Can you work these out from the model? Positions are in its coordinate system, mm. Face numbers are marked on the shaded views. Give positions to 0.01 mm unless a question says otherwise; leave off trailing zeros. Write each loop counter-clockwise with the first axis right and the second up, starting at its lowest first coordinate (ties: lowest second). Pieces come first, ordered by that corner, then holes. Notation, with made-up numbers: (-20.5, 64) -> (22.5, 64) arc R27 cw to (22.5, 102) -> close; hole circle Ø9 at (-18, -18). An arc over 180 degrees is marked (long way). Answer as CSV lines item,"result". Start each with the question number.
1. I'm going to push flat-ended pins straight in: P1, Ø1, axis at y = -1.5, z = -4, coming from the +X side; P2, Ø2.5, axis at x = 7, y = -5.5, coming from the +Z side. Where does each tip first touch, or does it pass through?
2. If we section it at D-D on x = 8.5: Write out the boundary of the cut face in (y, z), plus the area to 3 significant figures.
3. If we section it at A-A on z = -13: Write out the boundary of the cut face in (x, y).
4. If we section it at B-B on x = -6.5: Write out the boundary of the cut face in (y, z).
5. If we mould it in two halves opening along Y, with no side actions, what happens to the marked faces 1, 2, 3 and 4? For each: pulls with the +Y half, pulls with the -Y half, needs draft (parallel to the pull), parting line crosses it, or undercut.
6. I need wall thicknesses on line 1 (Z direction, x = -4.5, y = -2.5); line 2 (Z direction, x = -1.75, y = -1.25); line 3 (X direction, y = -7.25, z = 10). Which ranges of each line are inside material? Lowest first, please. Write a range as [from, to].
7. If we section it at C-C on x = 2.75: Write out the boundary of the cut face in (y, z).
```python
from build123d import *

# Parameters (mm, degrees)
F0_W      = 22.75429
F0_H      = 42.548669
F1_DEPTH  = 9.398
F2_R      = 2.54
F4_DEPTH  = 0.508
F6_DEPTH  = 1.9812
F7_R      = 3.013325
F8_DEPTH  = 1.9812
F9_R      = 2.713026
F10_DEPTH = 1.0414
F11_R     = 1.117074
F12_DEPTH = 0.5588
F13_R     = 2.450394
F14_DEPTH = 1.1176
F15_R     = 1.193925
F16_DEPTH = 0.6604


with BuildPart() as f1:
    # F0 (on Front) → F1 (new body)
    with BuildSketch(Plane.XZ):
        with Locations((1.757446, -0.647479)):
            Rectangle(F0_W, F0_H)
    extrude(amount=F1_DEPTH)

    # F2
    f2_edges = [f1.edges().sort_by_distance(p)[0] for p in [
        (13.134591, -9.398, -0.647479),
        (-9.619699, -9.398, -0.647479),
        (13.134591, 0, -0.647479),
        (-9.619699, 0, -0.647479),
    ]]
    fillet(f2_edges, radius=F2_R)

    # F3 (on face) → F4 (cut)
    with BuildSketch(Plane.XY.offset(20.626856)):
        with BuildLine():
            Line((9.49368, -0.802048), (-5.928423, -0.802048))
            ThreePointArc((-5.928423, -0.802048), (-7.724474, -1.545997), (-8.468423, -3.342048))
            Line((-8.468423, -3.342048), (-8.468423, -6.049972))
            ThreePointArc((-8.468423, -6.049972), (-7.724474, -7.846024), (-5.928423, -8.589972))
            Line((-5.928423, -8.589972), (9.49368, -8.589972))
            ThreePointArc((9.49368, -8.589972), (11.289732, -7.846024), (12.03368, -6.049972))
            Line((12.03368, -6.049972), (12.03368, -3.342048))
            ThreePointArc((12.03368, -3.342048), (11.289732, -1.545997), (9.49368, -0.802048))
        make_face()
    extrude(amount=-F4_DEPTH, mode=Mode.SUBTRACT)

    # F5 (on face) → F6 (join)
    with BuildSketch(Plane.XY.offset(20.118856)):
        Polygon((9.422873, -2.225276), (6.099785, -2.225276), (4.438241, -5.103154), (6.099785, -7.981033), (9.422873, -7.981033), (11.084417, -5.103154), align=None)
    extrude(amount=F6_DEPTH)

    # F7 (on face) → F8 (join)
    with BuildSketch(Plane.XY.offset(20.118856)):
        with Locations((-4.526955, -4.731211)):
            Circle(F7_R)
    extrude(amount=F8_DEPTH)

    # F9 (on face) → F10 (cut)
    with BuildSketch(Plane.XY.offset(22.100056)):
        with Locations((-4.526955, -4.731211)):
            Circle(F9_R)
    extrude(amount=-F10_DEPTH, mode=Mode.SUBTRACT)

    # F11 (on face) → F12 (join)
    with BuildSketch(Plane.XY.offset(21.058656)):
        with Locations((-4.526955, -4.731211)):
            Circle(F11_R)
    extrude(amount=F12_DEPTH)

    # F13 (on face) → F14 (cut)
    with BuildSketch(Plane.XY.offset(22.100056)):
        with Locations((7.78931, -5.203744)):
            Circle(F13_R)
    extrude(amount=-F14_DEPTH, mode=Mode.SUBTRACT)

    # F15 (on face) → F16 (join)
    with BuildSketch(Plane.XY.offset(20.982456)):
        with Locations((7.78931, -5.203744)):
            Circle(F15_R)
    extrude(amount=F16_DEPTH)


solid = f1.part
```
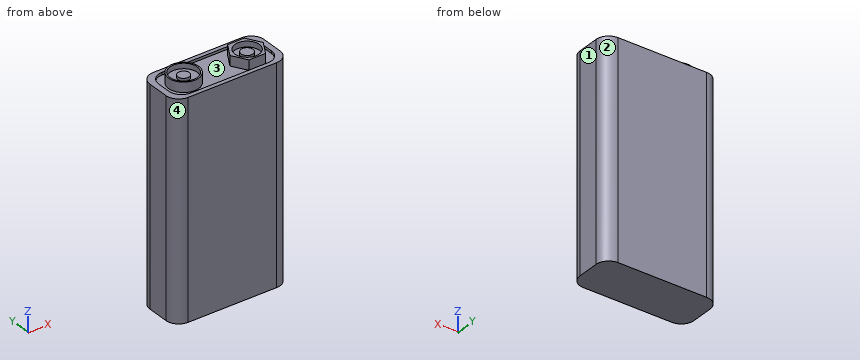
Computed values:
1,P1,"stops at x = 13.08"
1,P2,"stops at z = 21.64"
2,outline,"(-9.4, -21.92) -> (0, -21.92) -> (0, 20.63) -> (-0.8, 20.63) -> (-0.8, 20.12) -> (-2.23, 20.12) -> (-2.23, 22.1) -> (-2.86, 22.1) -> (-2.86, 20.98) -> (-4.24, 20.98) -> (-4.24, 21.64) -> (-6.16, 21.64) -> (-6.16, 20.98) -> (-7.55, 20.98) -> (-7.55, 22.1) -> (-7.98, 22.1) -> (-7.98, 20.12) -> (-8.59, 20.12) -> (-8.59, 20.63) -> (-9.4, 20.63) -> close"
2,area,"403 mm2"
3,outline,"(-9.62, -6.86) arc R2.54 ccw to (-7.08, -9.4) -> (10.59, -9.4) arc R2.54 ccw to (13.13, -6.86) -> (13.13, -2.54) arc R2.54 ccw to (10.59, 0) -> (-7.08, 0) arc R2.54 ccw to (-9.62, -2.54) -> close"
4,outline,"(-9.4, -21.92) -> (0, -21.92) -> (0, 20.63) -> (-0.87, 20.63) -> (-0.87, 20.12) -> (-2.45, 20.12) -> (-2.45, 22.1) -> (-2.87, 22.1) -> (-2.87, 21.06) -> (-6.59, 21.06) -> (-6.59, 22.1) -> (-7.01, 22.1) -> (-7.01, 20.12) -> (-8.52, 20.12) -> (-8.52, 20.63) -> (-9.4, 20.63) -> close"
5,face 1,"needs draft"
5,face 2,"pulls with the +Y half"
5,face 3,"undercut"
5,face 4,"pulls with the -Y half"
6,line 1,"z = [-21.92, 21.06]"
6,line 2,"z = [-21.92, 20.12]"
6,line 3,"x = [-9.59, 13.1]"
7,outline,"(-9.4, -21.92) -> (0, -21.92) -> (0, 20.63) -> (-0.8, 20.63) -> (-0.8, 20.12) -> (-8.59, 20.12) -> (-8.59, 20.63) -> (-9.4, 20.63) -> close"
